Answer from the drawing. Dimensions are ordinates in mm from the lowest x, y and z of the part. Round coordinates to 2 decimals unless told otherwise and drop trailing zeros. Loops run counter-clockwise (first coordinate to the right, second up) from the corner with the lowest first, then second, coordinate; pieces in that order, holes last. Notation, with made-up numbers: M -30.5,28 L 20.5,28 A34 ccw 20.5,60 Z; hole C 12,42 d2. An arc over 180 degrees is marked long. Answer as a JSON object with one key per item and string values.
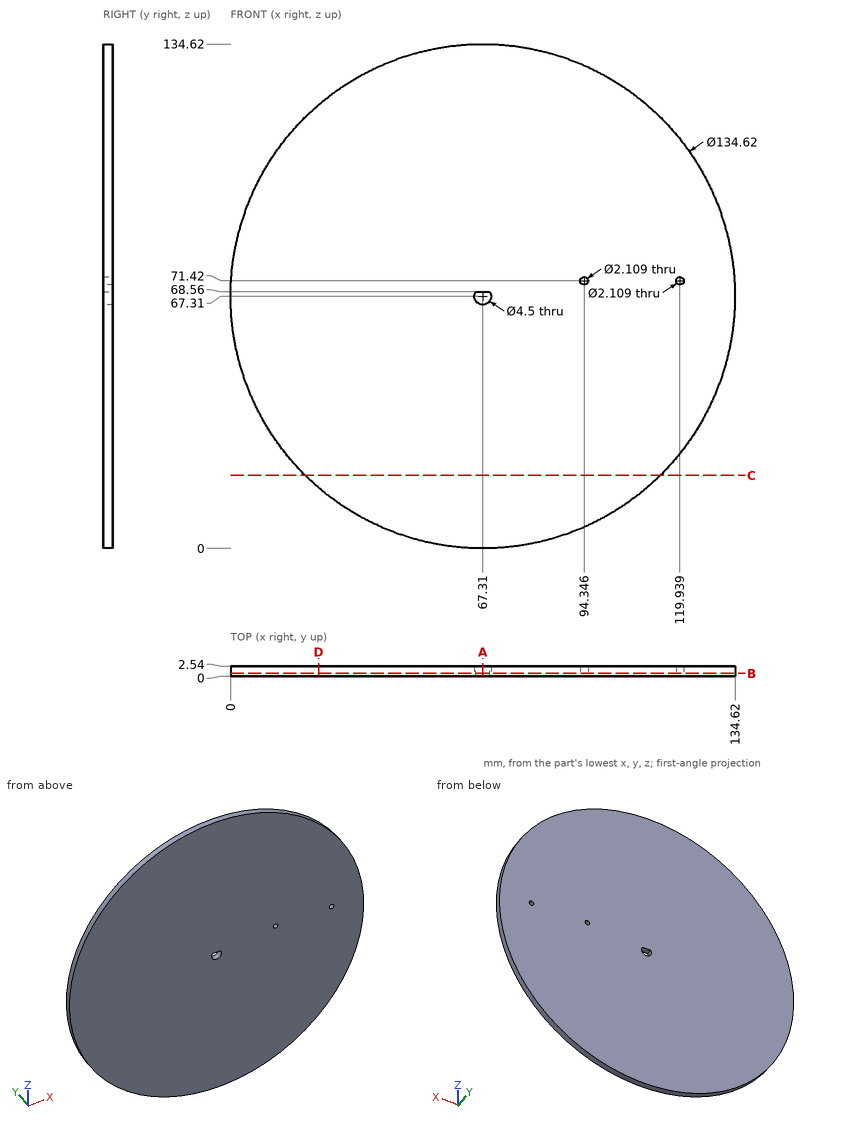
Item 1: The part is cut by section A-A (x = 67.31). Give the vertices of the cut face in (y, z), then the cut area to 3 significant figures.
Values follow:
{"outline": "M 0,0 L 2.54,0 L 2.54,65.06 L 0,65.06 Z; M 0,68.56 L 2.54,68.56 L 2.54,134.62 L 0,134.62 Z", "area": "333 mm^2"}
Item 2: The part is cut by section C-C (z = 19.5). Give the vertices of the cut face in (x, y).
Values follow:
{"outline": "M 19.93,0 L 114.69,0 L 114.69,2.54 L 19.93,2.54 Z"}
Item 3: The part is cut by section B-B (y = 0.7). Give the number of separate pieces and of enclosed holes in the cut face, then the cut area to 3 significant figures.
Values follow:
{"separate pieces": "1", "enclosed holes": "3", "area": "14,200 mm^2"}
Item 4: The part is cut by section D-D (x = 23.5). Give the vertices of the cut face in (y, z).
Values follow:
{"outline": "M 0,16.21 L 2.54,16.21 L 2.54,118.41 L 0,118.41 Z"}
Item 5: Straight lines are drawn through the part: line 1 (X direction, y = 1.45, z = 67.31); line 2 (X direction, y = 2.35, z = 71) (1 decimal); line 3 (Z direction, x = 65.5, y = 0.15) (1 decimal). For each, find the intervals that lie inside material, in ascending order.
Values follow:
{"line 1": "0 to 65.06, 69.56 to 134.62", "line 2": "0.1 to 93.4, 95.3 to 119, 120.9 to 134.5", "line 3": "0 to 66, 68.6 to 134.6"}
Item 6: A flat-ended cylindrical pin translates along its axis: P1, Ø1, axis at y = 1, z = 33, coming from the -X side. Find the tip coordinate at first contact, or state that the pin passes through.
Values follow:
{"P1": "x = 9.11"}
